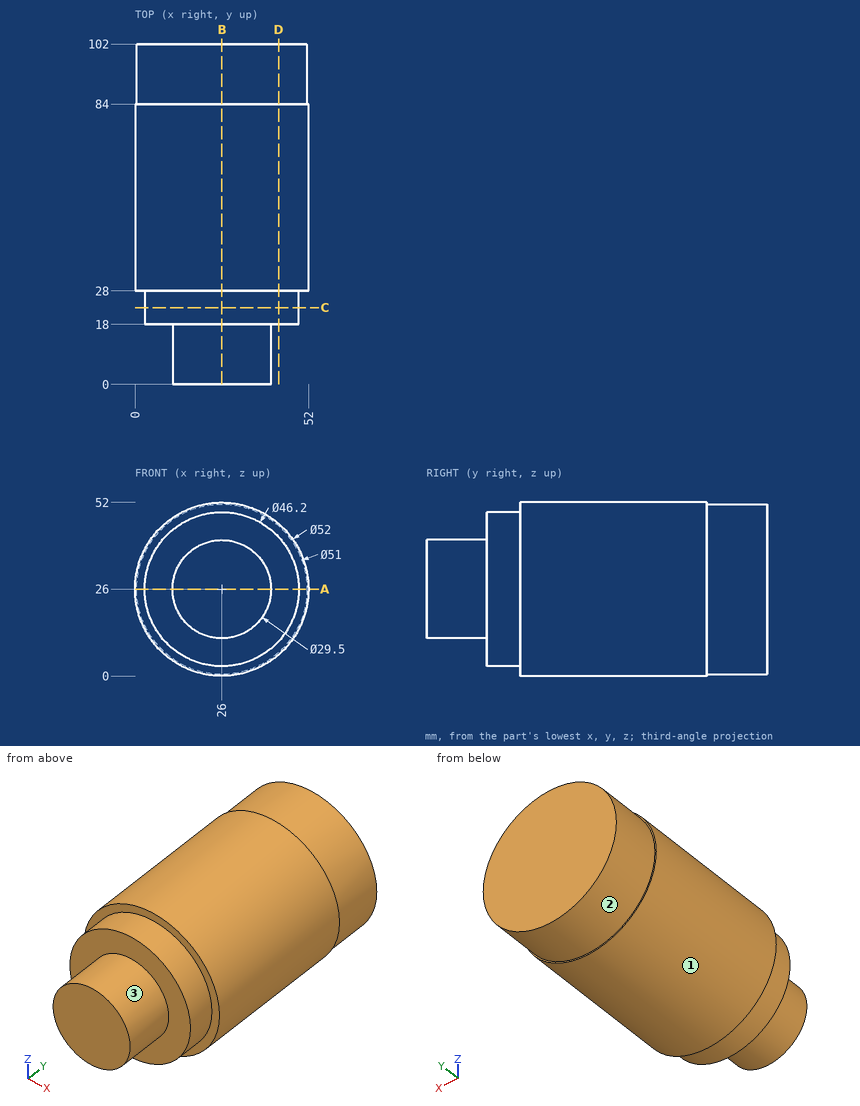
Geometry: see drawing. Coordinates: mm, zero at the bounding-box minimum. A direction names the side the tool comes from. Give positions to 0.01 mm unless a question says otherwise; leave off trailing zeros. Loops run counter-clockwise (first coordinate to the right, second up) from the corner with the lowest first, then second, coordinate; pieces in that order, holes last. Notation, with made-up numbers: (44, -12.75) -> (50, -12.75) arc R10 ccw to (50, 6.25) -> close; hole circle Ø10 at (85, -15.5). An arc over 180 degrees is marked (long way). Answer as a JSON object with one key per item and string values. Group by question number.
Item 1: Pin query (flat end, axial travel): P1, Ø12, axis at y = 71, z = 40.5, coming from the -X side; P2, Ø1.5, axis at x = 28, y = 14, coming from the +Z side; P3, Ø8, axis at x = 29.5, y = 78.5, coming from the +Z side. Return the tip coordinate at first contact, or that it passes through.
Item 2: Line query: probe 1 along Y at (x, z) = (27, 6.5); probe 2 along Z at (x, y) = (26.5, 43); probe 3 along Y at (x, z) = (3.5, 20). Output: solid intervals per line, ascending.
Item 3: Cut plane A-A, the plane z = 26. Return the cut outline in (x, y), and give its area (3 significant figures).
Item 4: Reachability of the marked faces 1, 2 and 3 from +Z, -Z, +X, -X, +Y, -Y: full face, straight path, thin tool, end or side. Return the list, or none.
Item 5: Cut plane B-B, the plane x = 26. Return the cut outline in (y, z), and give its area (3 significant figures).
Item 6: Cut plane D-D, the plane x = 43. Return the cut outline in (y, z), and give its area (3 significant figures).
Item 7: Cut plane C-C, the plane y = 23. Return the cut outline in (x, z).
Checks:
{
 "1": {"P1": "stops at x = 1.43", "P2": "stops at z = 40.7", "P3": "stops at z = 52"},
 "2": {"probe 1": "y = 18 to 102", "probe 2": "z = 0 to 52", "probe 3": "y = 28 to 102"},
 "3": {"outline": "(0, 28) -> (2.9, 28) -> (2.9, 18) -> (11.25, 18) -> (11.25, 0) -> (40.75, 0) -> (40.75, 18) -> (49.1, 18) -> (49.1, 28) -> (52, 28) -> (52, 84) -> (51.5, 84) -> (51.5, 102) -> (0.5, 102) -> (0.5, 84) -> (0, 84) -> close", "area": "4,820 mm²"},
 "4": {"face 1": "+Y, -Y", "face 2": "+Y", "face 3": "-Y"},
 "5": {"outline": "(0, 11.25) -> (18, 11.25) -> (18, 2.9) -> (28, 2.9) -> (28, 0) -> (84, 0) -> (84, 0.5) -> (102, 0.5) -> (102, 51.5) -> (84, 51.5) -> (84, 52) -> (28, 52) -> (28, 49.1) -> (18, 49.1) -> (18, 40.75) -> (0, 40.75) -> close", "area": "4,820 mm²"},
 "6": {"outline": "(18, 10.36) -> (28, 10.36) -> (28, 6.33) -> (84, 6.33) -> (84, 6.99) -> (102, 6.99) -> (102, 45.01) -> (84, 45.01) -> (84, 45.67) -> (28, 45.67) -> (28, 41.64) -> (18, 41.64) -> close", "area": "3,200 mm²"},
 "7": {"outline": "circle Ø46.2 at (26, 26)"}
}
